from build123d import *

# Parameters (mm, degrees)
F0_R     = 11.0363
F1_DEPTH = 6.985


with BuildPart() as f1:
    # F0 (on Top) → F1 (new body)
    with BuildSketch(Plane.XY):
        with BuildLine():
            ThreePointArc((12.7707550595, 28.4936086172), (13.2626459449, 30.5424816606), (13.4279664867, 32.6430783639))
            ThreePointArc((13.4279664867, 32.6430783639), (11.9644057547, 38.739247563), (7.8927606994, 43.5065314296))
            ThreePointArc((7.8927606994, 43.5065314296), (-4.13e-08, 46.0710448506), (-7.8927607663, 43.506531381))
            ThreePointArc((-7.8927607663, 43.506531381), (-12.7707550555, 36.7925481229), (-12.7707550095, 28.4936084631))
            ThreePointArc((-12.7707550095, 28.4936084631), (8.1e-08, 19.2151118771), (12.7707550595, 28.4936086172))
        make_face()
        with Locations((0, 32.6430783639)):
            Circle(F0_R, mode=Mode.SUBTRACT)
        with BuildLine():
            ThreePointArc((7.8927606994, 43.5065314296), (11.9644057547, 38.739247563), (13.4279664867, 32.6430783639))
            ThreePointArc((13.4279664867, 32.6430783639), (13.2626459449, 30.5424816606), (12.7707550595, 28.4936086172))
            Line((12.7707550595, 28.4936086172), (15.7855213384, 37.772105162))
            Line((15.7855213384, 37.772105162), (7.8927606994, 43.5065314296))
        make_face()
        with BuildLine():
            ThreePointArc((-7.8927607663, 43.506531381), (-4.13e-08, 46.0710448506), (7.8927606994, 43.5065314296))
            Line((7.8927606994, 43.5065314296), (0, 49.2409577411))
            Line((0, 49.2409577411), (-7.8927607663, 43.506531381))
        make_face()
        with BuildLine():
            Line((11.5032957401, 24.5927699357), (12.7707550595, 28.4936086172))
            ThreePointArc((12.7707550595, 28.4936086172), (8.1e-08, 19.2151118771), (-12.7707550095, 28.4936084631))
            Line((-12.7707550095, 28.4936084631), (-11.5032957401, 24.5927699357))
            ThreePointArc((-11.5032957401, 24.5927699357), (-10.9512854258, 19.3407426236), (-12.583190869, 14.3182541071))
            Line((-12.583190869, 14.3182541071), (-18.6915672291, 3.7382358996))
            ThreePointArc((-18.6915672291, 3.7382358996), (-22.225217153, -0.1862799289), (-27.0496113837, -2.3342386297))
            Line((-27.0496113837, -2.3342386297), (-31.0615663455, -3.1870059819))
            ThreePointArc((-31.0615663455, -3.1870059819), (-19.8192420037, -5.8860492535), (-14.8417686341, -16.3215391819))
            ThreePointArc((-14.8417686341, -16.3215391819), (-15.7336484589, -21.1336920446), (-18.2908113758, -25.306602613))
            Line((-18.2908113758, -25.306602613), (-15.5463156437, -22.258531306))
            ThreePointArc((-15.5463156437, -22.258531306), (-11.2739317272, -19.1544626947), (-6.1083763601, -18.0564900067))
            Line((-6.1083763601, -18.0564900067), (6.1083763601, -18.0564900067))
            ThreePointArc((6.1083763601, -18.0564900067), (11.2739317272, -19.1544626947), (15.5463156437, -22.258531306))
            Line((15.5463156437, -22.258531306), (18.2908113758, -25.306602613))
            ThreePointArc((18.2908113758, -25.306602613), (16.6407750687, -9.607555858), (31.0615666162, -3.1870060395))
            Line((31.0615666162, -3.1870060395), (27.0496113837, -2.3342386297))
            ThreePointArc((27.0496113837, -2.3342386297), (22.225217153, -0.1862799289), (18.6915672291, 3.7382358996))
            Line((18.6915672291, 3.7382358996), (12.583190869, 14.3182541071))
            ThreePointArc((12.583190869, 14.3182541071), (10.9512854258, 19.3407426236), (11.5032957401, 24.5927699357))
        make_face()
        Circle(F0_R, mode=Mode.SUBTRACT)
        with BuildLine():
            ThreePointArc((-12.7707550095, 28.4936084631), (-12.7707550555, 36.7925481229), (-7.8927607663, 43.506531381))
            Line((-7.8927607663, 43.506531381), (-15.7855213384, 37.772105162))
            Line((-15.7855213384, 37.772105162), (-12.7707550095, 28.4936084631))
        make_face()
        with BuildLine():
            Line((40.6043632939, -5.21539009), (31.0615666162, -3.1870060395))
            ThreePointArc((31.0615666162, -3.1870060395), (38.2486591322, -7.3364760466), (41.6241418349, -14.9179347913))
            Line((41.6241418349, -14.9179347913), (40.6043632939, -5.21539009))
        make_face()
        with BuildLine():
            ThreePointArc((41.6241418349, -14.9179347913), (38.2486591322, -7.3364760466), (31.0615666162, -3.1870060395))
            ThreePointArc((31.0615666162, -3.1870060395), (16.6407750687, -9.607555858), (18.2908113758, -25.306602613))
            ThreePointArc((18.2908113758, -25.306602613), (25.4779040103, -29.4560724062), (33.7313812405, -28.5885969234))
            ThreePointArc((33.7313812405, -28.5885969234), (39.5313754327, -23.6349338421), (41.6977016076, -16.3215391819))
            ThreePointArc((41.6977016076, -16.3215391819), (41.6792990544, -15.6187738716), (41.6241418349, -14.9179347913))
        make_face()
        with Locations((28.2697351208, -16.3215391819)):
            Circle(F0_R, mode=Mode.SUBTRACT)
        with BuildLine():
            ThreePointArc((-14.8417686341, -16.3215391819), (-19.8192420037, -5.8860492535), (-31.0615663455, -3.1870059819))
            ThreePointArc((-31.0615663455, -3.1870059819), (-38.2486589518, -7.3364758463), (-41.6241418074, -14.9179345303))
            ThreePointArc((-41.6241418074, -14.9179345303), (-39.8986951958, -23.0355224663), (-33.7313810924, -28.5885969893))
            ThreePointArc((-33.7313810924, -28.5885969893), (-25.477903931, -29.4560723893), (-18.2908113758, -25.306602613))
            ThreePointArc((-18.2908113758, -25.306602613), (-15.7336484589, -21.1336920446), (-14.8417686341, -16.3215391819))
        make_face()
        with Locations((-28.2697351208, -16.3215391819)):
            Circle(F0_R, mode=Mode.SUBTRACT)
        with BuildLine():
            ThreePointArc((-41.6241418074, -14.9179345303), (-38.2486589518, -7.3364758463), (-31.0615663455, -3.1870059819))
            Line((-31.0615663455, -3.1870059819), (-40.6043632939, -5.21539009))
            Line((-40.6043632939, -5.21539009), (-41.6241418074, -14.9179345303))
        make_face()
        with BuildLine():
            Line((42.6439203104, -24.6204788705), (41.6241418349, -14.9179347913))
            ThreePointArc((41.6241418349, -14.9179347913), (41.6792990544, -15.6187738716), (41.6977016076, -16.3215391819))
            ThreePointArc((41.6977016076, -16.3215391819), (39.5313754327, -23.6349338421), (33.7313812405, -28.5885969234))
            Line((33.7313812405, -28.5885969234), (42.6439203104, -24.6204788705))
        make_face()
        with BuildLine():
            ThreePointArc((33.7313812405, -28.5885969234), (25.4779040103, -29.4560724062), (18.2908113758, -25.306602613))
            Line((18.2908113758, -25.306602613), (24.8188419555, -32.556715072))
            Line((24.8188419555, -32.556715072), (33.7313812405, -28.5885969234))
        make_face()
        with BuildLine():
            ThreePointArc((-33.7313810924, -28.5885969893), (-39.8986951958, -23.0355224663), (-41.6241418074, -14.9179345303))
            Line((-41.6241418074, -14.9179345303), (-42.6439203104, -24.6204788705))
            Line((-42.6439203104, -24.6204788705), (-33.7313810924, -28.5885969893))
        make_face()
        with BuildLine():
            Line((-24.8188419555, -32.556715072), (-18.2908113758, -25.306602613))
            ThreePointArc((-18.2908113758, -25.306602613), (-25.477903931, -29.4560723893), (-33.7313810924, -28.5885969893))
            Line((-33.7313810924, -28.5885969893), (-24.8188419555, -32.556715072))
        make_face()
    extrude(amount=F1_DEPTH)


solid = f1.part
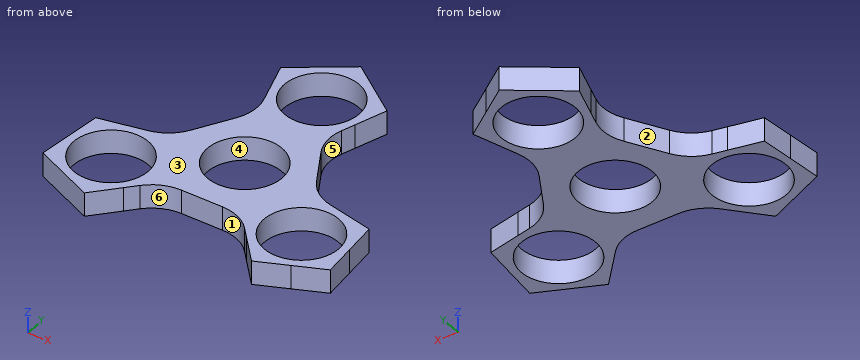
Can you work these out from the model? Positions are in its coordinate system, mm. Face numbers are marked on the shaded views. A direction names the side the tool comes from. Coordinates: 2 decimals unless noted, no trailing zeros. Write each loop counter-clockwise with the first axis right and the second up, starting at its lowest first coordinate (ties: lowest second). Pieces come first, ordered by that corner, then holes. Notation, with made-up numbers: (33, 13.5) -> (41, 13.5) arc R21 cw to (41, 52.5) -> close; hole circle Ø10 at (69, 54.5). An arc over 180 degrees is marked (long way). Write each question's results on one line, items separated by ' | '. Start each with the question number.
Q1. Imagine slicing it at A-A (y = 42.5). Write out the boundary of the cut face in (x, z) (3 decimals), then the cut area to 3 significant figures.
Q2. Imagine slicing it at C-C (y = 0). Write out the boundary of the cut face in (x, z) (3 decimals), then the cut area to 3 significant figures.
Q3. Imagine slicing it at B-B (y = -12.5). Write out the boundary of the cut face in (x, z) (3 decimals).
Q4. I'm going to push flat-ended pins straight in: pin 1 (2 mm diameter, centred on x = 2, z = 4.5, fed in from -Y); pin 2 (1.5 mm diameter, centred on x = 31.5, z = 5, fed in from -Y); pin 3 (1 mm diameter, centred on x = -10, z = 1.5, fed in from +Y). Where does each tip first touch, or does it pass through?
Q5. We'd pull the mould along X, two halves only. Please class the marked faces 1, 2, 3 and 4: +X half, -X half, draft (parallel to the pull), parting line (faces both ways), or undercut.
Q6. On a 3-axis mill with a long thin cutter (end or side, diameter ignored), from which of +Z, -Z, +X, -X, +Y, -Y can I reach the whole of each face in a straight line? I mean the marked faces 5 and 6. Say none if no direction works.
Q7. Imagine slicing it at D-D (z = 1.75). Write out the boundary of the cut face in (x, y), then the cut area to 3 significant figures.
Q8. If I drill on probe 1 along Y at (x, z) = (0, 5.5); probe 2 along X at (y, z) = (-14, 1); probe 3 along Y at (x, z) = (3, 6.75), over which ranges is the centre line in solid material (lowest first)?
Taken from the geometry:
1) outline: (-9.278, 0) -> (-4.964, 0) -> (-4.964, 6.985) -> (-9.278, 6.985) -> close; (4.964, 0) -> (9.278, 0) -> (9.278, 6.985) -> (4.964, 6.985) -> close | area: 60.3 mm^2
2) outline: (-21.975, 0) -> (-11.036, 0) -> (-11.036, 6.985) -> (-21.975, 6.985) -> close; (11.036, 0) -> (21.975, 0) -> (21.975, 6.985) -> (11.036, 6.985) -> close | area: 153 mm^2
3) outline: (-41.37, 0) -> (-38.623, 0) -> (-38.623, 6.985) -> (-41.37, 6.985) -> close; (-17.916, 0) -> (17.916, 0) -> (17.916, 6.985) -> (-17.916, 6.985) -> close; (38.623, 0) -> (41.37, 0) -> (41.37, 6.985) -> (38.623, 6.985) -> close
4) pin 1: stops at y = -18.06 | pin 2: stops at y = -29.92 | pin 3: stops at y = 42.34
5) face 1: undercut | face 2: -X half | face 3: draft | face 4: undercut
6) face 5: +Z, -Z, +X | face 6: +Z, -Z, -Y
7) outline: (-42.64, -24.62) -> (-24.82, -32.56) -> (-15.55, -22.26) arc R12.7 cw to (-6.11, -18.06) -> (6.11, -18.06) arc R12.7 cw to (15.55, -22.26) -> (24.82, -32.56) -> (42.64, -24.62) -> (40.6, -5.22) -> (27.05, -2.33) arc R12.7 cw to (18.69, 3.74) -> (12.58, 14.32) arc R12.7 cw to (11.5, 24.59) -> (15.79, 37.77) -> (0, 49.24) -> (-15.79, 37.77) -> (-11.5, 24.59) arc R12.7 cw to (-12.58, 14.32) -> (-18.69, 3.74) arc R12.7 cw to (-27.05, -2.33) -> (-40.6, -5.22) -> close; hole circle Ø22.07 at (-28.27, -16.32); hole circle Ø22.07 at (0, 0); hole circle Ø22.07 at (0, 32.64); hole circle Ø22.07 at (28.27, -16.32) | area: 1,660 mm^2
8) probe 1: y = -18.06 to -11.04, 11.04 to 21.61, 43.68 to 49.24 | probe 2: x = -41.53 to -39.06, -17.48 to 17.48, 39.06 to 41.53 | probe 3: y = -18.06 to -10.62, 10.62 to 22.02, 43.26 to 47.06
